from build123d import *

# Parameters (mm, degrees)
F1_DEPTH = 25.4
F3_DEPTH = 12.7
F5_DEPTH = 13.716


with BuildPart() as f1:
    # F0 (on Front) → F1 (new body)
    with BuildSketch(Plane.XZ):
        Polygon((0, 19.05), (0, 0), (57.15, 0), (57.15, 19.05), (44.45, 19.05), (44.45, 5.132193), (6.35, 5.132193), (6.35, 19.05), align=None)
    extrude(amount=F1_DEPTH)

    # F2 (on face) → F3 (cut)
    with BuildSketch(Plane.XY.offset(19.05)):
        Polygon((44.45, 0), (44.45, -25.4), (57.15, -17.763132), (57.15, 0), align=None)
    extrude(amount=-F3_DEPTH, mode=Mode.SUBTRACT)

    # F4 (on face) → F5 (join)
    with BuildSketch(Plane.XY.offset(5.132193)):
        Polygon((6.35, 0), (6.35, -15.941272), (16.244914, 0), align=None)
    extrude(amount=F5_DEPTH)


solid = f1.part
Geometry check sheet. Reference: the model listing, model coordinates, mm. A direction names the side the tool comes from. Give positions to 0.01 mm unless a question says otherwise; leave off trailing zeros. Write each loop counter-clockwise with the first axis right and the second up, starting at its lowest first coordinate (ties: lowest second). Pieces come first, ordered by that corner, then holes. Notation, with made-up numbers: M 26.5,-33 L 60.5,-33 A30 cw 60.5,1 Z; hole C -36,17 d3. An arc over 180 degrees is marked long. One line per question, with ' | ' between items.
1. Cross-section at B-B (y = -16.5). Enter the section's corners in (x, z), plus the area to 3 significant figures.
Ans:
outline: M 0,0 L 57.15,0 L 57.15,6.35 L 44.45,6.35 L 44.45,5.13 L 6.35,5.13 L 6.35,19.05 L 0,19.05 Z | area: 397 mm2
2. Set-up check for faces 1 (the face through (10, -6, 18.848)), 2 (the face through (51, -10, 6.35)), 3 (the face through (6.35, -20, 13)): record each of +Z, -Z, +X, -X, +Y, -Y from which the full face is reachable in a straight line by a thin tool's end or side.
Ans:
face 1: +Z, +X, +Y, -Y | face 2: +Z, +Y | face 3: +Z, -Y
3. Scan lines: line 1 along Z through (x, y) = (38, -20); line 2 along X through (y, z) = (-16.5, 10.5); line 3 along X through (y, z) = (-23.5, 16.75). Record each from-to range of solid material in increasing order. Write a range as from..to.
Ans:
line 1: 0..5.13 | line 2: 0..6.35 | line 3: 0..6.35, 47.61..57.15
4. Gauge pin test, flat end, axial feed: pin 1 (4 mm diameter, centred on x = 24.5, y = -22.5, fed in from +Z). Record the tip position at first contact, or that the pin passes through.
Ans:
pin 1: z = 5.13
5. Cross-section at D-D (y = -8.5). Enter the section's corners in (x, z).
Ans:
outline: M 0,0 L 57.15,0 L 57.15,6.35 L 44.45,6.35 L 44.45,5.13 L 10.97,5.13 L 10.97,18.85 L 6.35,18.85 L 6.35,19.05 L 0,19.05 Z
6. Mould release check, pull along X, two halves, no side actions. Record for faces 4 (the face through (57.15, -15, 5)), 5 (the face through (3, -13, 19.05)), 6 (the face through (44.45, -13, 6)), 7 (the face through (50.711, -21.635, 12.789)): released by +X, released by -X, zero draft, split by the parting line, or undercut.
Ans:
face 4: released by +X | face 5: zero draft | face 6: undercut | face 7: undercut
7. Cross-section at C-C (x = 26). Enter the section's corners in (y, z).
Ans:
outline: M -25.4,0 L 0,0 L 0,5.13 L -25.4,5.13 Z
8. Cross-section at A-A (z = 13.5). Enter the section's corners in (x, y).
Ans:
outline: M 0,-25.4 L 6.35,-25.4 L 6.35,-15.94 L 16.24,0 L 0,0 Z; M 44.45,-25.4 L 57.15,-25.4 L 57.15,-17.76 Z
